Geometry: final body of the model. Coordinates: model frame, mm. Face numbers are marked on the shaded views. A direction names the side the tool comes from. Give positions to 0.01 mm unless a question says otherwise; leave off trailing zeros. Loops run counter-clockwise (first coordinate to the right, second up) from the corner with the lowest first, then second, coordinate; pieces in that order, holes last. Notation, with made-up numbers: (23.25, 76) - (74.25, 76) arc R34 cw to (74.25, 114) - close; hole circle Ø2 at (85, -28.75). An arc over 180 degrees is marked (long way). Use CSV: the item, a comma, the result in double quotes. Start each with the question number.
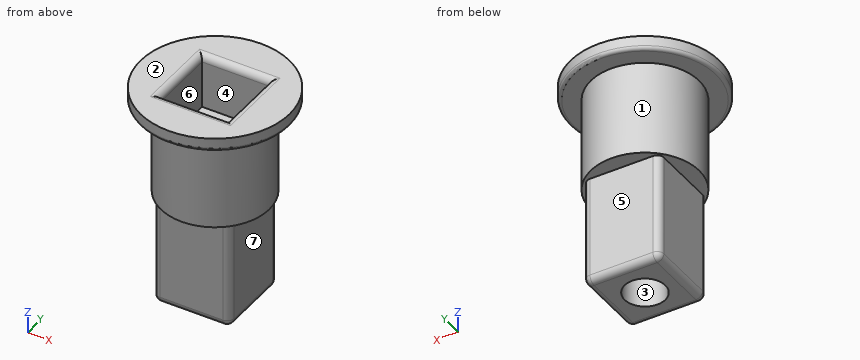
```python
from build123d import *

# Parameters (mm, degrees)
ESQUISSE1_R      = 4
EXTRUSION1_DEPTH = 7
ESQUISSE3_W      = 5.65685425
ESQUISSE3_H      = 5.65685425
EXTRUSION3_DEPTH = 8
CONG_4_R         = 0.5
ESQUISSE7_R      = 5.5
EXTRUSION6_DEPTH = 1
ESQUISSE8_R      = 1.5
EXTRUSION7_DEPTH = 18.790446875
ESQUISSE9_W      = 4.949747468
ESQUISSE9_H      = 4.949747468
EXTRUSION8_DEPTH = 4
CONG_5_R         = 0.25
CONG_6_R         = 0.5


with BuildPart() as part:
    # Esquisse1 → Extrusion1 (new body)
    with BuildSketch(Plane.XY):
        Circle(ESQUISSE1_R)
    extrude(amount=-EXTRUSION1_DEPTH)

    # Esquisse3 → Extrusion3 (add)
    with BuildSketch(Plane(origin=(0, 0, -7), x_dir=(-1, 0, 0), z_dir=(0, 0, -1))):
        Rectangle(ESQUISSE3_W, ESQUISSE3_H)
    extrude(amount=EXTRUSION3_DEPTH)

    # Congé4
    cong_4_edges = [part.edges().sort_by_distance(p)[0] for p in [
        (-2.828427125, 0, -15),
        (0, 2.828427125, -15),
        (2.828427125, 2.828427125, -11),
        (2.828427125, -2.828427125, -11),
        (-2.828427125, -2.828427125, -11),
        (-2.828427125, 2.828427125, -11),
        (2.828427125, 0, -15),
        (0, -2.828427125, -15),
    ]]
    fillet(cong_4_edges, radius=CONG_4_R)

    # Esquisse7 → Extrusion6 (add)
    with BuildSketch(Plane.XY):
        Circle(ESQUISSE7_R)
    extrude(amount=EXTRUSION6_DEPTH)

    # Esquisse8 → Extrusion7 (cut, through all)
    with BuildSketch(Plane.XY.offset(1)):
        Circle(ESQUISSE8_R)
    extrude(amount=-EXTRUSION7_DEPTH, mode=Mode.SUBTRACT)

    # Esquisse9 → Extrusion8 (cut)
    with BuildSketch(Plane.XY.offset(1)):
        Rectangle(ESQUISSE9_W, ESQUISSE9_H)
    extrude(amount=-EXTRUSION8_DEPTH, mode=Mode.SUBTRACT)

    # Congé5
    cong_5_edges = [part.edges().sort_by_distance(p)[0] for p in [
        (-5.5, 0, 0),
    ]]
    fillet(cong_5_edges, radius=CONG_5_R)

    # Congé6
    cong_6_edges = [part.edges().sort_by_distance(p)[0] for p in [
        (-2.474873734, 0, 1),
        (0, -2.474873734, 1),
        (2.474873734, 0, 1),
        (0, 2.474873734, 1),
    ]]
    fillet(cong_6_edges, radius=CONG_6_R)


solid = part.part
```
Item 1: Section A-A (z = -11.75). Output: boundary loops of the cut face in (x, y), plus the area to 3 significant figures.
Item 2: Mould query, pull axis X, two halves, no side actions, for the marked faces 1, 2, 3 and 4. Classes: pulls with the +X half, pulls with the -X half, needs draft (parallel to the pull), parting line crosses it, or undercut.
Item 3: Reachability of the marked faces 5, 6 and 7 from +Z, -Z, +X, -X, +Y, -Y: full face, straight path, thin tool, end or side. Return the list, or none.
Item 4: Ray query, probe 1 along Y at (x, z) = (0, -9.5); probe 2 along X at (y, z) = (-1.25, -1.5); probe 3 along Z at (x, y) = (1, 4.25). Return the intervals inside material, ascending.
Item 5: Section D-D (z = -1.5). Output: boundary loops of the cut face in (x, y).
Item 6: Pin query (flat end, axial travel): pin 1 Ø4 at (x, y) = (0, 0) entering from +Z; pin 2 Ø5 at (x, z) = (-1.5, -3) entering from -Y; pin 3 Ø1.4 at (y, z) = (-1, -11.5) entering from -X. Return the tip coordinate at first contact, or that it passes through.
Item 7: Section B-B (y = 0). Output: boundary loops of the cut face in (x, z).
Outcome:
1,outline,"(-2.83, -2.33) arc R0.5 ccw to (-2.33, -2.83) - (2.33, -2.83) arc R0.5 ccw to (2.83, -2.33) - (2.83, 2.33) arc R0.5 ccw to (2.33, 2.83) - (-2.33, 2.83) arc R0.5 ccw to (-2.83, 2.33) - close; hole circle Ø3 at (0, 0)"
1,area,"24.7 mm2"
2,face 1,"parting line crosses it"
2,face 2,"needs draft"
2,face 3,"undercut"
2,face 4,"undercut"
3,face 5,"-Z, +X, -X, +Y"
3,face 6,"+Z"
3,face 7,"-Z, +X, +Y, -Y"
4,probe 1,"y = -2.83 to -1.5, 1.5 to 2.83"
4,probe 2,"x = -3.8 to -2.47, 2.47 to 3.8"
4,probe 3,"z = 0 to 1"
5,outline,"circle Ø8 at (0, 0); hole (-2.47, -2.47) - (2.47, -2.47) - (2.47, 2.47) - (-2.47, 2.47) - close"
6,pin 1,"stops at z = -3"
6,pin 2,"stops at y = -4"
6,pin 3,"stops at x = -2.83"
7,outline,"(-5.5, 0.25) arc R0.25 ccw to (-5.25, 0) - (-4, 0) - (-4, -7) - (-2.83, -7) - (-2.83, -14.5) arc R0.5 ccw to (-2.33, -15) - (-1.5, -15) - (-1.5, -3) - (-2.47, -3) - (-2.47, 0.5) arc R0.5 ccw to (-2.97, 1) - (-5.5, 1) - close; (1.5, -15) - (2.33, -15) arc R0.5 ccw to (2.83, -14.5) - (2.83, -7) - (4, -7) - (4, 0) - (5.25, 0) arc R0.25 ccw to (5.5, 0.25) - (5.5, 1) - (2.97, 1) arc R0.5 ccw to (2.47, 0.5) - (2.47, -3) - (1.5, -3) - close"
